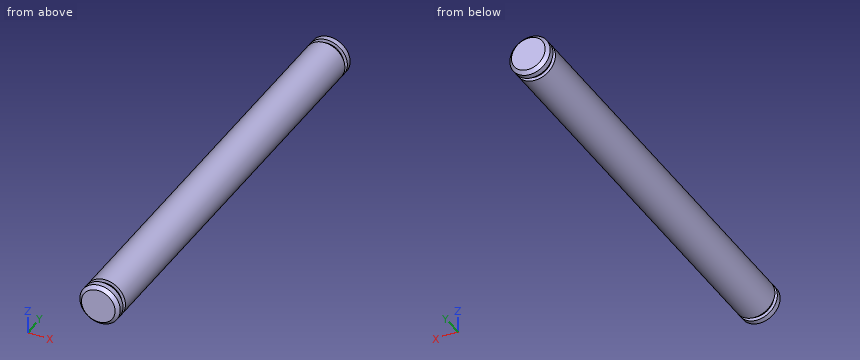
```python
from build123d import *

# Parameters (mm, degrees)
SKETCH1_R          = 3
EXTRUDE_50_DEPTH   = 66.5
CUT_EXTRUDE1_START = -2
SKETCH2_R          = 3
SKETCH2_R_2        = 2.5
CUT_EXTRUDE1_DEPTH = 0.7
CUT_EXTRUDE2_START = -1.3
SKETCH3_R          = 3
SKETCH3_R_2        = 2.5
CUT_EXTRUDE2_DEPTH = 0.7
CHAMFER1_SIZE      = 0.5


with BuildPart() as part:
    # Sketch1 → Extrude 50 (new body)
    with BuildSketch(Plane(origin=(0, 0, 0), x_dir=(1, 0, 0), z_dir=(0, 1, 0))):
        with Locations(Location((0, 0, 0), (0, 0, 270))):
            Circle(SKETCH1_R)
    extrude(amount=EXTRUDE_50_DEPTH)

    # Sketch2 → Cut-Extrude1 (cut)
    with BuildSketch(Plane(origin=(0, 66.5, 0), x_dir=(1, 0, 0), z_dir=(0, 1, 0)).offset(CUT_EXTRUDE1_START)):
        with Locations(Location((0, 0, 0), (0, 0, 270))):
            Circle(SKETCH2_R)
        with Locations(Location((0, 0, 0), (0, 0, 270))):
            Circle(SKETCH2_R_2, mode=Mode.SUBTRACT)
    extrude(amount=CUT_EXTRUDE1_DEPTH, mode=Mode.SUBTRACT)

    # Sketch3 → Cut-Extrude2 (cut)
    with BuildSketch(Plane.XZ.offset(CUT_EXTRUDE2_START)):
        with Locations(Location((0, 0, 0), (0, 0, 270))):
            Circle(SKETCH3_R)
        with Locations(Location((0, 0, 0), (0, 0, 90))):
            Circle(SKETCH3_R_2, mode=Mode.SUBTRACT)
    extrude(amount=-CUT_EXTRUDE2_DEPTH, mode=Mode.SUBTRACT)

    # Chamfer1
    chamfer1_edges = [part.edges().sort_by_distance(p)[0] for p in [
        (0, 0, -3),
        (0, 66.5, -3),
    ]]
    chamfer(chamfer1_edges, length=CHAMFER1_SIZE)


solid = part.part
```
Check sheet for the modelled part. Datum: model origin and axes. Units: mm. Coordinates: 2 decimals unless noted, no trailing zeros. Loops run counter-clockwise (first coordinate to the right, second up) from the corner with the lowest first, then second, coordinate; pieces in that order, holes last. Notation, with made-up numbers: M -24,4.25 L -2,4.25 A5 cw -2,9.25 Z; hole C 40,-7.75 d1. An arc over 180 degrees is marked long. Answer as a JSON object with one key per item and string values.
1. Depth check by flat-ended pin: P1, Ø1.5, axis at y = 36, z = 2, coming from the -X side. Enter the tip coordinate at first touch or a pass-through.
Outcome:
{"P1": "x = -2.73"}
2. Sectioned sample at A-A on y = 36.5. Record the cut outline in (x, z), and give its area (3 significant figures).
Outcome:
{"outline": "C 0,0 d6", "area": "28.3 mm²"}
3. Scan lines: L1, parallel to Y at x = -1.7, z = -1.9; L2, parallel to X at y = 62, z = 0.15; L3, parallel to Y at x = -0.65, z = -2.6. Record each from-to range of solid material in increasing order. Write a range as from..to.
Outcome:
{"L1": "0.05..1.3, 2..64.5, 65.2..66.45", "L2": "-3..3", "L3": "0.18..1.3, 2..64.5, 65.2..66.32"}
